Model file for the job. Use its own axes, mm. A direction names the side the tool comes from. Round coordinates to 2 decimals unless told otherwise and drop trailing zeros. Write each loop counter-clockwise with the first axis right and the second up, starting at its lowest first coordinate (ties: lowest second). Pieces come first, ordered by that corner, then holes. Notation, with made-up numbers: (53.5, 22) - (91.5, 22) arc R10 ccw to (91.5, 26) - close; hole circle Ø9 at (47.25, 79.25). An arc over 180 degrees is marked (long way). Answer as a JSON object with one key per item and string values. Group by question number.
from build123d import *

# Parameters (mm, degrees)
SKETCH_2_R      = 20
EXTRUDE_1_DEPTH = 200


with BuildPart() as part:
    # 草图1 → 旋转1 (revolve)
    with BuildSketch(Plane.XY, mode=Mode.PRIVATE) as revolve_1_sk:
        with BuildLine():
            Line((0, 288.881257919), (0, 0))
            Line((0, 0), (20, 0))
            Line((20, 0), (20, 100))
            Line((20, 100), (15, 100))
            Line((15, 100), (15, 200))
            Line((15, 200), (465, 200))
            Line((465, 200), (465, 240))
            Line((465, 240), (15, 240))
            Line((15, 240), (15, 290))
            ThreePointArc((15, 290), (7.520830803, 289.161331306), (0, 288.881257919))
        make_face()
        with BuildLine():
            Line((0, 390), (0, 290))
            Line((0, 290), (15, 290))
            ThreePointArc((15, 290), (76.6217369, 324.014324021), (101.118742081, 390))
            ThreePointArc((101.118742081, 390), (71.50174823, 461.50174823), (0, 491.118742081))
            Line((0, 491.118742081), (0, 390))
        make_face()
        with BuildLine():
            Line((0, 290), (0, 288.881257919))
            ThreePointArc((0, 288.881257919), (7.520830803, 289.161331306), (15, 290))
            Line((15, 290), (0, 290))
        make_face()
    revolve(revolve_1_sk.sketch.rotate(Axis((0, 290, 0), (0, 1, 0)), 90), axis=Axis((0, 290, 0), (0, 1, 0)))

    # 草图2 → 凸台-拉伸1 (add)
    with BuildSketch(Plane.XZ):
        with Locations(Location((0, 0, 0), (0, 0, 270))):
            Circle(SKETCH_2_R)
    extrude(amount=EXTRUDE_1_DEPTH)


solid = part.part
(1) Slice it at C-C (y = -100.5). Write the cut outline in (x, z).
(2) Slice it at D-D (y = 182.5). Write the cut outline in (x, z).
(3) Pull direction Y, two halves, no side cores. Call faces 3 (the flat face through (0, -200, 0)), 4 (the cylindrical face through (-19.524, -47.9, 4.336)), 5 (the cylindrical face through (-12.65, 265.35, -8.06)): pulls with the +Y half, pulls with the -Y half, needs draft (parallel to the pull), parting line crosses it, or undercut.
(4) Slice it at A-A (z = 0). Write the cut outline in (x, y).
(5) 3-axis set-ups, long thin cutter, end or side, ignore diameter. For faces 1 (the cylindrical face through (453.942, 220.28, 100.803)), 2 (the flat face through (-15, 100, -3)): which of +Z, -Z, +X, -X, +Y, -Y reach the whole face in a straight line?
(6) Slice it at B-B (x = 0). Write the cut outline in (y, z), then the cut area to 3 significant figures.
(7) Flat gauge pins, fed straight in: pin 1 (12 mm diameter, centred on x = -6.5, z = 8, fed in from +Y); pin 2 (12 mm diameter, centred on x = -188.5, z = 8.5, fed in from +Y). Where does each tip first touch, or does it go through?
(8) Drill centre lines: line 1 (Y direction, x = 153, z = -409.5); line 2 (Y direction, x = -27.5, z = 48.5); line 3 (Y direction, x = 36, z = 84). Where is each one in solid material? Low to high. Write a range as from..to.
Answer:
{
 "1": {"outline": "circle Ø40 at (0, 0)"},
 "2": {"outline": "circle Ø30 at (0, 0)"},
 "3": {"face 3": "pulls with the -Y half", "face 4": "needs draft", "face 5": "undercut"},
 "4": {"outline": "(-465, 200) - (-15, 200) - (-15, 100) - (-20, 100) - (-20, -200) - (20, -200) - (20, 100) - (15, 100) - (15, 200) - (465, 200) - (465, 240) - (15, 240) - (15, 290) arc R101.12 ccw (long way) to (-15, 290) - (-15, 240) - (-465, 240) - close"},
 "5": {"face 1": "+Y, -Y", "face 2": "none"},
 "6": {"outline": "(-200, -20) - (100, -20) - (100, -15) - (200, -15) - (200, -465) - (240, -465) - (240, -15) - (290, -15) arc R101.12 ccw (long way) to (290, 15) - (240, 15) - (240, 465) - (200, 465) - (200, 15) - (100, 15) - (100, 20) - (-200, 20) - close", "area": "85,800 mm²"},
 "7": {"pin 1": "y = 491.03", "pin 2": "y = 240"},
 "8": {"line 1": "200..240", "line 2": "200..240, 305.64..474.36", "line 3": "200..240, 346.72..433.28"}
}
